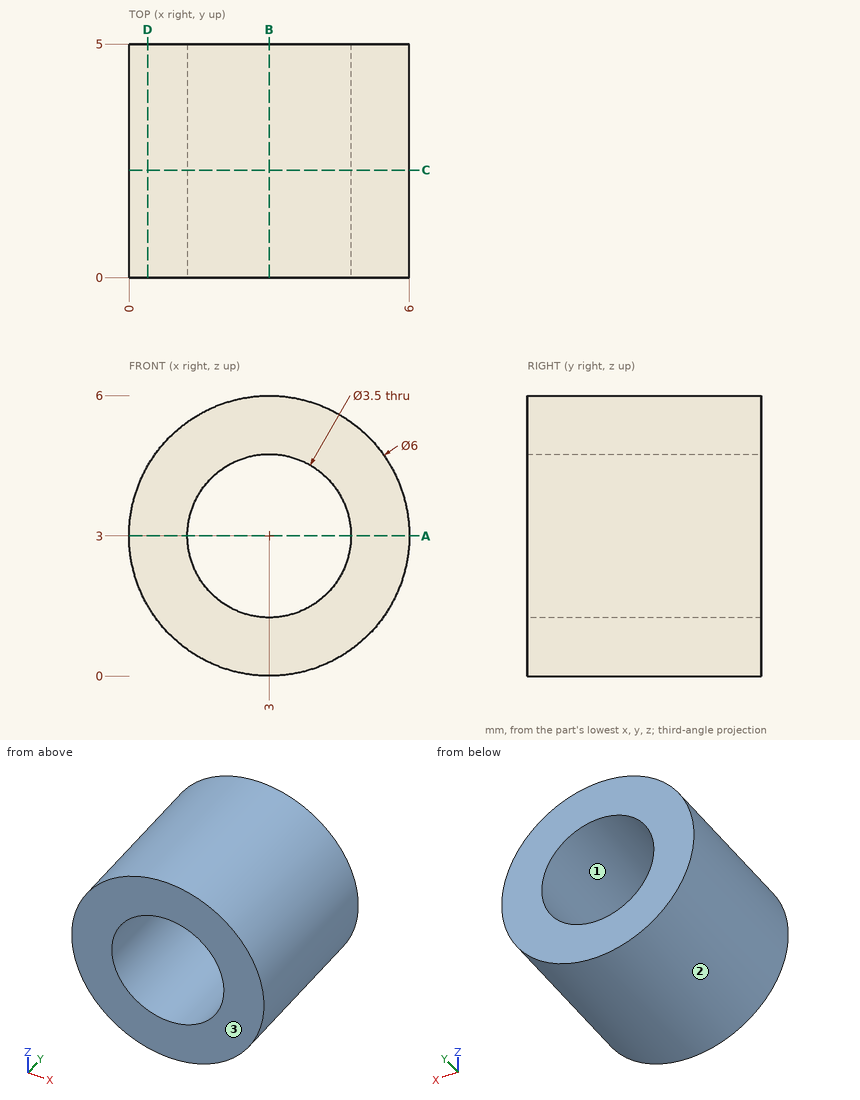
Design review of the part shown in the three views and the two pictorial views. Dimensions are in mm from the part's minimum x, y and z. Coordinates: 2 decimals unless noted, no trailing zeros. Write each loop counter-clockwise with the first axis right and the second up, starting at its lowest first coordinate (ties: lowest second). Pieces come first, ordered by that corner, then holes. Notation, with made-up numbers: (-24, 67) - (28, 67) arc R18 cw to (28, 91) - close; hole circle Ø3 at (30, 31). An arc over 180 degrees is marked (long way). Write item = value, one per line.
(1) Consider section A-A, the plane z = 3. Give the boundary of the cut face in (x, y).
Result sheet:
outline = (0, 0) - (1.25, 0) - (1.25, 5) - (0, 5) - close; (4.75, 0) - (6, 0) - (6, 5) - (4.75, 5) - close
(2) For P1, Ø2, axis at y = 4.5, z = 3.5, coming from the +X side; P2, Ø2, axis at x = 3, z = 3, coming from the -Y side; P3, Ø1.5, axis at x = 1.5, y = 0.5, coming from the +Z side; P4, Ø2, axis at x = 1, y = 2.5, coming from the -Z side, all flat-tipped, find the tip position at first contact; note any pin that passes through.
Result sheet:
P1 = 6
P2 = through
P3 = 5.9
P4 = 0.17
(3) Consider section D-D, the plane x = 0.4. Give the boundary of the cut face in (y, z).
Result sheet:
outline = (0, 1.5) - (5, 1.5) - (5, 4.5) - (0, 4.5) - close
(4) Consider section C-C, the plane y = 2.3. Give the boundary of the cut face in (x, z), then the cut area to 3 significant figures.
Result sheet:
outline = circle Ø6 at (3, 3); hole circle Ø3.5 at (3, 3)
area = 18.7 mm^2
(5) Mouldability with a two-part tool opening along X and no side actions: class the marked faces 1, 2 and 3 as pulls with the +X half, pulls with the -X half, needs draft (parallel to the pull), parting line crosses it, or undercut.
Result sheet:
face_1 = undercut
face_2 = parting line crosses it
face_3 = needs draft
(6) For line 1 (X direction, y = 3.3, z = 3); line 2 (Z direction, x = 2.4, y = 1.6); line 3 (X direction, y = 0.25, z = 3.75), list the stretches that pass through material, from the lowest coordinate up. Write a range as [from, to].
Result sheet:
line_1 = [0, 1.25], [4.75, 6]
line_2 = [0.06, 1.36], [4.64, 5.94]
line_3 = [0.1, 1.42], [4.58, 5.9]
(7) Consider section B-B, the plane x = 3. Give the boundary of the cut face in (y, z), then the cut area to 3 significant figures.
Result sheet:
outline = (0, 0) - (5, 0) - (5, 1.25) - (0, 1.25) - close; (0, 4.75) - (5, 4.75) - (5, 6) - (0, 6) - close
area = 12.5 mm^2
